Could you check a few things on this model? Use its own coordinates, in mm. Face numbers are marked on the shaded views. A direction names the side the tool comes from. Give positions to 0.01 mm unless a question says otherwise; leave off trailing zeros. Order: outer loops, then holes, each group sorted by start corner. A loop starts at its lowest first (then second) coordinate and runs counter-clockwise, first axis right, second up. Notation, with made-up numbers: M -4,-39.5 L 53,-39.5 A16 cw 53,-30.5 Z; hole C 55,-11 d2. An arc over 180 degrees is marked long. Use a Markdown table: item, result. Add a question column.
```python
from build123d import *

# Parameters (mm, degrees)
CROQUIS1_W                 = 54.3
CROQUIS1_H                 = 59
CROQUIS1_W_2               = 50.3
CROQUIS1_H_2               = 55
SALIENTE_EXTRUIR1_DEPTH    = 24
CROQUIS2_W                 = 54.3
CROQUIS2_H                 = 59
SALIENTE_EXTRUIR2_DEPTH    = 2
CORTAR_EXTRUIR4_DEPTH      = 54.3
CORTAR_EXTRUIR5_REACH      = 81.601
CROQUIS7_W                 = 5.111111111
CROQUIS7_H                 = 51
CROQUIS7_W_2               = 5.111111112
CORTAR_EXTRUIR6_DEPTH      = 66.864425147
CORTAR_EXTRUIR6_DEPTH_BACK = 66.864425147
CROQUIS8_R                 = 6.65
CORTAR_EXTRUIR7_DEPTH      = 66.864425147
CORTAR_EXTRUIR7_DEPTH_BACK = 66.864425147
CROQUIS9_R                 = 2.5
CROQUIS10_W                = 3
CROQUIS10_H                = 2
SALIENTE_EXTRUIR3_DEPTH    = 24
REDONDEO1_R                = 10


with BuildPart() as part:
    # Croquis1 → Saliente-Extruir1 (new body)
    with BuildSketch(Plane(origin=(0, 0, 0), x_dir=(1, 0, 0), z_dir=(0, 1, 0))):
        with Locations((-25.15, -27.5)):
            Rectangle(CROQUIS1_W, CROQUIS1_H)
        with Locations((-25.15, -27.5)):
            Rectangle(CROQUIS1_W_2, CROQUIS1_H_2, mode=Mode.SUBTRACT)
    extrude(amount=SALIENTE_EXTRUIR1_DEPTH)

    # Croquis2 → Saliente-Extruir2 (add)
    with BuildSketch(Plane.XZ):
        with Locations((-25.15, 27.5)):
            Rectangle(CROQUIS2_W, CROQUIS2_H)
    extrude(amount=SALIENTE_EXTRUIR2_DEPTH)

    # Croquis6 → Cortar-Extruir4 (cut)
    with BuildSketch(Plane.ZY.offset(52.3)):
        Polygon((55, 24), (55, 0), (55, -2), (57, -2), (57, 24), align=None)
    extrude(amount=-CORTAR_EXTRUIR4_DEPTH, mode=Mode.SUBTRACT)

    # Croquis7 → Cortar-Extruir5 (cut, up to next)
    with BuildSketch(Plane(origin=(0, 0, 0), x_dir=(1, 0, 0), z_dir=(0, 1, 0)), mode=Mode.PRIVATE) as cortar_extruir5_sk1:
        with Locations((-45.744444445, -27.5)):
            Rectangle(CROQUIS7_W, CROQUIS7_H)
    cortar_extruir5_tool1 = extrude(cortar_extruir5_sk1.sketch, amount=-CORTAR_EXTRUIR5_REACH, mode=Mode.PRIVATE) & part.part
    # Croquis7 → Cortar-Extruir5 (cut, up to next)
    with BuildSketch(Plane(origin=(0, 0, 0), x_dir=(1, 0, 0), z_dir=(0, 1, 0)), mode=Mode.PRIVATE) as cortar_extruir5_sk2:
        with Locations((-35.522222223, -27.5)):
            Rectangle(CROQUIS7_W, CROQUIS7_H)
    cortar_extruir5_tool2 = extrude(cortar_extruir5_sk2.sketch, amount=-CORTAR_EXTRUIR5_REACH, mode=Mode.PRIVATE) & part.part
    # Croquis7 → Cortar-Extruir5 (cut, up to next)
    with BuildSketch(Plane(origin=(0, 0, 0), x_dir=(1, 0, 0), z_dir=(0, 1, 0)), mode=Mode.PRIVATE) as cortar_extruir5_sk3:
        with Locations((-25.3, -27.5)):
            Rectangle(CROQUIS7_W_2, CROQUIS7_H)
    cortar_extruir5_tool3 = extrude(cortar_extruir5_sk3.sketch, amount=-CORTAR_EXTRUIR5_REACH, mode=Mode.PRIVATE) & part.part
    # Croquis7 → Cortar-Extruir5 (cut, up to next)
    with BuildSketch(Plane(origin=(0, 0, 0), x_dir=(1, 0, 0), z_dir=(0, 1, 0)), mode=Mode.PRIVATE) as cortar_extruir5_sk4:
        with Locations((-15.077777777, -27.5)):
            Rectangle(CROQUIS7_W, CROQUIS7_H)
    cortar_extruir5_tool4 = extrude(cortar_extruir5_sk4.sketch, amount=-CORTAR_EXTRUIR5_REACH, mode=Mode.PRIVATE) & part.part
    # Croquis7 → Cortar-Extruir5 (cut, up to next)
    with BuildSketch(Plane(origin=(0, 0, 0), x_dir=(1, 0, 0), z_dir=(0, 1, 0)), mode=Mode.PRIVATE) as cortar_extruir5_sk5:
        with Locations((-4.855555556, -27.5)):
            Rectangle(CROQUIS7_W, CROQUIS7_H)
    cortar_extruir5_tool5 = extrude(cortar_extruir5_sk5.sketch, amount=-CORTAR_EXTRUIR5_REACH, mode=Mode.PRIVATE) & part.part
    add(cortar_extruir5_tool1.solids().sort_by_distance((-45.744444, 0, 27.5))[0], mode=Mode.SUBTRACT)
    add(cortar_extruir5_tool2.solids().sort_by_distance((-35.522222, 0, 27.5))[0], mode=Mode.SUBTRACT)
    add(cortar_extruir5_tool3.solids().sort_by_distance((-25.3, 0, 27.5))[0], mode=Mode.SUBTRACT)
    add(cortar_extruir5_tool4.solids().sort_by_distance((-15.077778, 0, 27.5))[0], mode=Mode.SUBTRACT)
    add(cortar_extruir5_tool5.solids().sort_by_distance((-4.855556, 0, 27.5))[0], mode=Mode.SUBTRACT)

    # Croquis8 → Cortar-Extruir6 (cut, two sides: drawn at the far end of the back side and taken through both)
    with BuildSketch(Plane(origin=(-25.15, 0, 0), x_dir=(0, 0, -1), z_dir=(1, 0, 0)).offset(-CORTAR_EXTRUIR6_DEPTH_BACK)):
        with Locations((-43, 15)):
            Circle(CROQUIS8_R)
    extrude(amount=CORTAR_EXTRUIR6_DEPTH + CORTAR_EXTRUIR6_DEPTH_BACK, mode=Mode.SUBTRACT)

    # Croquis9 → Cortar-Extruir7 (cut, two sides: drawn at the far end of the back side and taken through both)
    with BuildSketch(Plane(origin=(-25.15, 0, 0), x_dir=(0, 0, -1), z_dir=(1, 0, 0)).offset(-CORTAR_EXTRUIR7_DEPTH_BACK)):
        with Locations((-30.8, 19)):
            Circle(CROQUIS9_R)
        with Locations((-30.8, 5)):
            Circle(CROQUIS9_R)
    extrude(amount=CORTAR_EXTRUIR7_DEPTH + CORTAR_EXTRUIR7_DEPTH_BACK, mode=Mode.SUBTRACT)

    # Croquis10 → Saliente-Extruir3 (add)
    with BuildSketch(Plane(origin=(0, 24, 0), x_dir=(1, 0, 0), z_dir=(0, 1, 0))):
        with Locations((-48.8, -17.4)):
            Rectangle(CROQUIS10_W, CROQUIS10_H)
        with Locations((-48.8, -23)):
            Rectangle(CROQUIS10_W, CROQUIS10_H)
        with Locations((-1.5, -23)):
            Rectangle(CROQUIS10_W, CROQUIS10_H)
        with Locations((-1.5, -17.4)):
            Rectangle(CROQUIS10_W, CROQUIS10_H)
    extrude(amount=-SALIENTE_EXTRUIR3_DEPTH)

    # Redondeo1
    # the kernel refuses this fillet: 10 mm, written as the material it takes off along each edge
    with BuildSketch(Plane(origin=(-3, 0, 7.211012025), x_dir=(0, 1, 0), z_dir=(0, 0, 1)), Plane(origin=(-3, 0, 12.811012025), x_dir=(0, 1, 0), z_dir=(0, 0, 1))) as redondeo1_piece_1:
        with BuildLine():
            CenterArc((3.67559519, -10), REDONDEO1_R, 90, 21.565185015)
            Line((0, -0.7), (-0.073511904, -0.514))
            ThreePointArc((-0.073511904, -0.514), (-0.2, -0.35), (-0.2, 0))
            Line((-0.2, 0), (0, 0.2))
            Line((0, 0.2), (3.67559519, 0.2))
            Line((3.67559519, 0.2), (3.67559519, 0))
        make_face()
    extrude(amount=20.377975949, mode=Mode.SUBTRACT)
    with BuildSketch(Plane(origin=(-47.3, 0, 29.297247359), x_dir=(0, 1, 0), z_dir=(0, 0, -1)), Plane(origin=(-47.3, 0, 34.897247359), x_dir=(0, 1, 0), z_dir=(0, 0, -1))) as redondeo1_piece_2:
        with BuildLine():
            CenterArc((4.358898944, -10), REDONDEO1_R, 90, 25.841932763)
            Line((0, -1), (-0.087177979, -0.82))
            ThreePointArc((-0.087177979, -0.82), (-0.2, -0.5), (-0.2, 0))
            Line((-0.2, 0), (0, 0.2))
            Line((0, 0.2), (4.358898944, 0.2))
            Line((4.358898944, 0.2), (4.358898944, 0))
        make_face()
    extrude(amount=23.794494718, mode=Mode.SUBTRACT)


solid = part.part
```
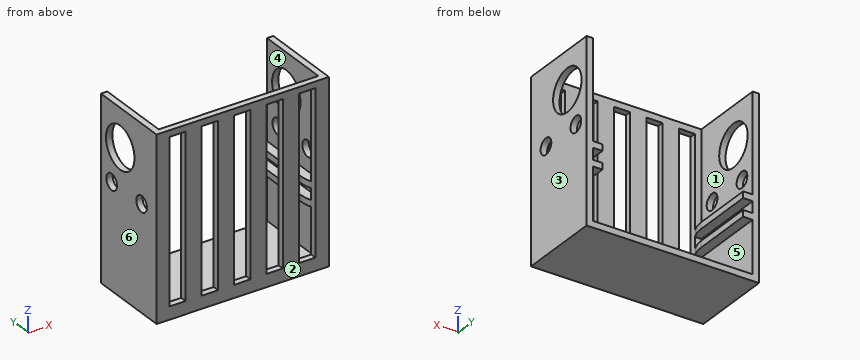
1) Suppose I cut it at A-A on x = -45.5. Please give me the cut outline in (y, z), and give its area (3 significant figures).
2) Suppose I cut it at C-C on z = 26.5. Please give me the cut outline in (x, y), and give its area (3 significant figures).
3) Suppose I cut it at B-B on y = 6.5. Count the separate pieces of the cut face and the enclosed holes in it, and give its area (3 significant figures).
4) We'd pull the mould along X, two halves only. Please class the marked faces 1, 2 and 3: pulls with the +X half, pulls with the -X half, needs draft (parallel to the pull), parting line crosses it, or undercut.
5) For pin 1 (1 mm diameter, centred on x = -4.5, y = 14, fed in from +Z); pin 2 (3 mm diameter, centred on x = -18.5, z = 35.5, fed in from +Y); pin 3 (2.5 mm diameter, centred on x = -49, y = 16, fed in from +Z); pin 4 (3.5 mm diameter, centred on x = -1, y = 16.5, fed in from +Z), each with a flat end and sliding along its axis, tell me the tip position at first contact or that it passes through.
6) For the marked faces 4, 5 and 6, which set-ups out of +Z, -Z, +X, -X, +Y, -Y let a thin tool reach every point of the face, with its end or its side?
7) Please list where these lines run through material, in increasing order: line 1 (Z direction, x = -0.5, y = 22); line 2 (Y direction, x = -51.5, z = 30.8); line 3 (X direction, y = 1, z = 50.5). Write a range as from..to.
Values found:
| question | item | result |
|---|---|---|
| 1 | outline | M -2,-2 L 24,-2 L 24,0 L 0,0 L 0,2 L -2,2 Z; M -2,53 L 0,53 L 0,55 L -2,55 Z |
| 1 | area | 60.0 mm^2 |
| 2 | outline | M -52.3,-2 L -48.3,-2 L -48.3,0 L -50.3,0 L -50.3,24 L -52.3,24 Z; M -43.19,-2 L -38.08,-2 L -38.08,0 L -43.19,0 Z; M -32.97,-2 L -27.86,-2 L -27.86,0 L -32.97,0 Z; M -22.74,-2 L -17.63,-2 L -17.63,0 L -22.74,0 Z; M -12.52,-2 L -7.41,-2 L -7.41,0 L -12.52,0 Z; M -2.3,-2 L 2,-2 L 2,24 L 0,24 L 0,0 L -2.3,0 Z |
| 2 | area | 153 mm^2 |
| 3 | separate pieces | 3 |
| 3 | enclosed holes | 0 |
| 3 | area | 337 mm^2 |
| 4 | face 1 | undercut |
| 4 | face 2 | needs draft |
| 4 | face 3 | pulls with the +X half |
| 5 | pin 1 | stops at z = 0 |
| 5 | pin 2 | stops at y = 0 |
| 5 | pin 3 | stops at z = 24 |
| 5 | pin 4 | stops at z = 55 |
| 6 | face 4 | +Z, +Y |
| 6 | face 5 | +Y |
| 6 | face 6 | +Z, -Z, -X, +Y, -Y |
| 7 | line 1 | z = -2..0, 16.4..18.4, 22..24 |
| 7 | line 2 | y = -2..2.5, 7.5..16.5, 21.5..24 |
| 7 | line 3 | x = -52.3..-50.3, 0..2 |
